Input: part model. Units: mm. Frame: model coordinates. A direction names the side the tool comes from. Round coordinates to 2 decimals unless told otherwise and drop trailing zeros. Write each loop counter-clockwise with the first axis right and the second up, starting at its lowest first coordinate (ties: lowest second). Pieces come first, ordered by that corner, then holes. Notation, with made-up numbers: (-23, -20.75) -> (21, -20.75) arc R29 cw to (21, 10.25) -> close; hole circle Ø8 at (3, -21.75). An arc over 180 degrees is marked (long way). Write item = value, one per line.
```python
from build123d import *

# Parameters (mm, degrees)
BOSS_EXTRUDE1_DEPTH = 25.4
SKETCH3_R           = 2.15265
CUT_EXTRUDE1_DEPTH  = 0.5
SKETCH2_R           = 2.25
BOSS_EXTRUDE2_DEPTH = 0.5
CUT_EXTRUDE2_DEPTH  = 0.5
FILLET2_R           = 38


with BuildPart() as part:
    # Sketch1 → Boss-Extrude1 (new body)
    with BuildSketch(Plane.XY):
        Polygon((-0.5, 0.5), (-53.34, 0.5), (-53.34, 0), (0, 0), (0, 75.78), (-76.50978813, 75.78), (-76.50978813, 75.28), (-0.5, 75.28), align=None)
    extrude(amount=BOSS_EXTRUDE1_DEPTH)

    # Sketch3 → Cut-Extrude1 (cut)
    with BuildSketch(Plane(origin=(0, 0, 0), x_dir=(-1, 0, 0), z_dir=(0, -1, 0))):
        with Locations(Location((50.16, -19.05, 0), (0, 0, 90))):
            Circle(SKETCH3_R)
        with Locations(Location((37.46, -19.05, 0), (0, 0, 90))):
            Circle(SKETCH3_R)
        with Locations(Location((24.76, -19.05, 0), (0, 0, 90))):
            Circle(SKETCH3_R)
        with Locations(Location((12.06, -19.05, 0), (0, 0, 90))):
            Circle(SKETCH3_R)
        with Locations(Location((37.46, -6.35, 0), (0, 0, 90))):
            Circle(SKETCH3_R)
        with Locations(Location((24.76, -6.35, 0), (0, 0, 90))):
            Circle(SKETCH3_R)
        with Locations(Location((12.06, -6.35, 0), (0, 0, 90))):
            Circle(SKETCH3_R)
        with Locations(Location((50.16, -6.35, 0), (0, 0, 90))):
            Circle(SKETCH3_R)
    extrude(amount=-CUT_EXTRUDE1_DEPTH, mode=Mode.SUBTRACT)

    # Sketch2 → Boss-Extrude2 (add)
    with BuildSketch(Plane(origin=(0, 75.78, 0), x_dir=(1, 0, 0), z_dir=(0, 1, 0))):
        with BuildLine():
            ThreePointArc((-38.00978813, -12.7), (-49.286177054, 14.523611076), (-76.50978813, 25.8))
            Line((-76.50978813, 25.8), (-76.50978813, 13.55))
            ThreePointArc((-76.50978813, 13.55), (-57.948235124, 5.861553006), (-50.25978813, -12.7))
            ThreePointArc((-50.25978813, -12.7), (-57.948235124, -31.261553006), (-76.50978813, -38.95))
            Line((-76.50978813, -38.95), (-76.50978813, -51.2))
            ThreePointArc((-76.50978813, -51.2), (-49.286177054, -39.923611076), (-38.00978813, -12.7))
        make_face()
        with Locations(Location((-63.689893146, -43.649964339, 0), (0, 0, 270))):
            Circle(SKETCH2_R, mode=Mode.SUBTRACT)
        with Locations((-45.559823791, -25.519894984)):
            Circle(SKETCH2_R, mode=Mode.SUBTRACT)
        with Locations((-45.559823791, 0.119894984)):
            Circle(SKETCH2_R, mode=Mode.SUBTRACT)
        with Locations(Location((-63.689893146, 18.249964339, 0), (0, 0, 270))):
            Circle(SKETCH2_R, mode=Mode.SUBTRACT)
    extrude(amount=-BOSS_EXTRUDE2_DEPTH)

    # Sketch2<3> → Cut-Extrude2 (cut)
    with BuildSketch(Plane(origin=(0, 75.78, 0), x_dir=(1, 0, 0), z_dir=(0, 1, 0))):
        with BuildLine():
            Line((-43.313020463, -25.4), (-47.806627118, -25.4))
            ThreePointArc((-47.806627118, -25.4), (-45.619792587, -27.769095674), (-43.309823791, -25.519894984))
            ThreePointArc((-43.309823791, -25.519894984), (-43.310623101, -25.459926188), (-43.313020463, -25.4))
        make_face()
        with BuildLine():
            ThreePointArc((-43.313020463, -25.4), (-45.559823791, -23.269894984), (-47.806627118, -25.4))
            Line((-47.806627118, -25.4), (-43.313020463, -25.4))
        make_face()
        with BuildLine():
            Line((-43.313020463, 0), (-47.806627118, 0))
            ThreePointArc((-47.806627118, 0), (-45.559823791, -2.130105016), (-43.313020463, 0))
        make_face()
        with BuildLine():
            ThreePointArc((-43.309823791, 0.119894984), (-45.619792587, 2.369095674), (-47.806627118, 0))
            Line((-47.806627118, 0), (-43.313020463, 0))
            ThreePointArc((-43.313020463, 0), (-43.310623101, 0.059926188), (-43.309823791, 0.119894984))
        make_face()
        with BuildLine():
            Line((-71.249275888, 0), (-76.50978813, -12.7))
            Line((-76.50978813, -12.7), (-76.50978813, -25.4))
            Line((-76.50978813, -25.4), (-53.536488411, -25.4))
            ThreePointArc((-53.536488411, -25.4), (-51.092160215, -19.257948702), (-50.25978813, -12.7))
            ThreePointArc((-50.25978813, -12.7), (-51.092160215, -6.142051298), (-53.536488411, 0))
            Line((-53.536488411, 0), (-71.249275888, 0))
        make_face()
        Polygon((-76.50978813, 0), (-76.50978813, -12.7), (-71.249275888, 0), align=None)
    extrude(amount=-CUT_EXTRUDE2_DEPTH, mode=Mode.SUBTRACT)

    # Fillet2
    fillet2_edges = [part.edges().sort_by_distance(p)[0] for p in [
        (-0.5, 75.28, 12.7),
        (0, 75.78, 12.7),
    ]]
    fillet(fillet2_edges, radius=FILLET2_R)


solid = part.part
```
1) First-contact query: P1, Ø0.6, axis at y = 0, z = 8.5, coming from the -X side; P2, Ø1, axis at y = 47, z = 12.5, coming from the -X side; P3, Ø4, axis at x = -63.69, z = -18.25, coming from the +Y side; P4, Ø5, axis at x = -12.06, z = 19.05, coming from the +Y side. Flat tips, straight axial feed; report the tip coordinate or a pass-through.
Solutions:
P1 = -53.34
P2 = -1.9
P3 = through
P4 = 67.69
2) Line query: L1, parallel to X at y = 0.1, z = 6.35; L2, parallel to Y at x = -44.5, z = 15.5; L3, parallel to X at y = 65, z = 8.5. Output: solid intervals per line, ascending. Write a range as from..to.
Solutions:
L1 = -53.34..-52.31, -48.01..-39.61, -35.31..-26.91, -22.61..-14.21, -9.91..0
L2 = 0..0.5, 75.28..75.78
L3 = -12.51..-11.48
3) Draft query along X for faces 4 (the face through (-35.326, 0.246, 6.63)), 5 (the face through (-48.026, 0.246, 6.63)), 6 (the face through (-27, 0.5, 13)), 7 (the face through (-11.927, 64.444, 12.878)). Return one class per face: +X half, -X half, draft (parallel to the pull), parting line (faces both ways), or undercut.
Solutions:
face_4 = undercut
face_5 = undercut
face_6 = draft
face_7 = -X half
4) Cut plane A-A (z = 6.35). Return the cut outline in (x, y).
Solutions:
outline = (-53.34, 0) -> (-52.31, 0) -> (-52.31, 0.5) -> (-53.34, 0.5) -> close; (-51.04, 75.28) -> (-38.5, 75.28) arc R38 cw to (-0.5, 37.28) -> (-0.5, 0.5) -> (-9.91, 0.5) -> (-9.91, 0) -> (0, 0) -> (0, 37.78) arc R38 ccw to (-38, 75.78) -> (-51.04, 75.78) -> close; (-48.01, 0) -> (-39.61, 0) -> (-39.61, 0.5) -> (-48.01, 0.5) -> close; (-35.31, 0) -> (-26.91, 0) -> (-26.91, 0.5) -> (-35.31, 0.5) -> close; (-22.61, 0) -> (-14.21, 0) -> (-14.21, 0.5) -> (-22.61, 0.5) -> close
5) Cut plane D-D (z = -11). Return the cut outline in (x, y), and give its area (3 significant figures).
Solutions:
outline = (-65.22, 75.28) -> (-46.17, 75.28) -> (-46.17, 75.78) -> (-65.22, 75.78) -> close
area = 9.53 mm^2
6) Access query for faces 1 (the face through (-65.686, 75.534, 44.688)), 2 (the face through (-14.16, 0.25, 6.82)), 3 (the face through (-49, 75.28, 12)). Directions: +Z, -Z, +X, -X, +Y, -Y. A direction counts if a zero-diameter tool reaches every point of the face in a straight line with its end or side. Return the directions, or none.
Solutions:
face_1 = +Y, -Y
face_2 = -Y
face_3 = +Z, -Z, -X
7) Cut plane C-C (y = 8). Return the cut outline in (x, z).
Solutions:
outline = (-0.5, 0) -> (0, 0) -> (0, 25.4) -> (-0.5, 25.4) -> close
